Part model, mm, in its own coordinate system. Coordinates: 2 decimals unless noted, no trailing zeros. Write each loop counter-clockwise with the first axis right and the second up, starting at its lowest first coordinate (ties: lowest second). Pieces come first, ordered by that corner, then holes. Notation, with made-up numbers: (68, 50.5) - (76, 50.5) arc R6 ccw to (76, 60.5) - close; hole circle Ø5 at (37.25, 5.5). An arc over 180 degrees is marked (long way). Use one line per item in the form item = value. Start each with the question number.
from build123d import *

# Parameters (mm, degrees)
SKETCH1_W           = 325
SKETCH1_H           = 5
BOSS_EXTRUDE1_DEPTH = 87
CHAMFER1_SIZE       = 60


with BuildPart() as part:
    # Sketch1 → Boss-Extrude1 (new body)
    with BuildSketch(Plane(origin=(0, 0, 0), x_dir=(1, 0, 0), z_dir=(0, 1, 0))):
        Rectangle(SKETCH1_W, SKETCH1_H)
    extrude(amount=BOSS_EXTRUDE1_DEPTH)

    # Chamfer1
    chamfer1_edges = [part.edges().sort_by_distance(p)[0] for p in [
        (162.5, 87, 0),
    ]]
    chamfer(chamfer1_edges, length=CHAMFER1_SIZE)


solid = part.part
Q1. Drill centre lines: probe 1 along X at (y, z) = (40.5, 1.95); probe 2 along X at (y, z) = (68, 1); probe 3 along Y at (x, z) = (145, 0). Where is each one in solid material? Low to high.
Q2. Slice it at B-B (x = 107). List the corners of the cut face in (y, z).
Q3. Slice it at C-C (y = 53). List the corners of the cut face in (x, z).
Q4. Slice it at A-A (z = 1.2). List the corners of the cut face in (x, y).
Solution:
q1.probe_1 = -162.5 to 149
q1.probe_2 = -162.5 to 121.5
q1.probe_3 = 0 to 44.5
q2.outline = (0, -2.5) - (82.5, -2.5) - (82.5, 2.5) - (0, 2.5) - close
q3.outline = (-162.5, -2.5) - (136.5, -2.5) - (136.5, 2.5) - (-162.5, 2.5) - close
q4.outline = (-162.5, 0) - (162.5, 0) - (162.5, 27) - (102.5, 87) - (-162.5, 87) - close
